```python
from build123d import *

# Parameters (mm, degrees)
BOX_W        = 100
BOX_H        = 32
BOX_DEPTH    = 52
SKETCH_W     = 100
SKETCH_H     = 25.7
POCKET_DEPTH = 5


with BuildPart() as part:
    # Box → Box (new body)
    with BuildSketch(Plane.XY):
        with Locations((50, 16)):
            Rectangle(BOX_W, BOX_H)
    extrude(amount=BOX_DEPTH)

    # Sketch → Pocket (cut)
    with BuildSketch(Plane.XZ):
        with Locations((50, 12.85)):
            Rectangle(SKETCH_W, SKETCH_H)
    extrude(amount=-POCKET_DEPTH, mode=Mode.SUBTRACT)


solid = part.part
```
Geometry: final body of the model. Coordinates: model frame, mm. A direction names the side the tool comes from. Coordinates: 2 decimals unless noted, no trailing zeros. Loops run counter-clockwise (first coordinate to the right, second up) from the corner with the lowest first, then second, coordinate; pieces in that order, holes last. Notation, with made-up numbers: (43, 29.5) -> (51, 29.5) arc R34 cw to (51, 59.5) -> close; hole circle Ø4 at (34, -21.5). An arc over 180 degrees is marked (long way). Use a Markdown table: item, result. Add a question column.
(1) Section query A-A, the plane x = 16. Return loops of the section in (y, z).
(2) Line query: line 1 along Z through (x, y) = (5, 3.5); line 2 along Y through (x, z) = (88, 5). Output: solid intervals per line, ascending.
(3) Pin query (flat end, axial travel): pin 1 Ø7.5 at (x, z) = (72.5, 11) entering from -Y. Return the tip coordinate at first contact, or that it passes through.
(4) Section query B-B, the plane z = 14.5. Return loops of the section in (x, y), plus the area to 3 significant figures.
(5) Access query for faces 1 (the flat face through (49, 5, 13)), 2 (the flat face through (49, 0, 39)). Directions: +Z, -Z, +X, -X, +Y, -Y. A direction counts if a zero-diameter tool reaches every point of the face in a straight line with its end or side. Return the directions, or none.
Answer:
| question | item | result |
|---|---|---|
| 1 | outline | (0, 25.7) -> (5, 25.7) -> (5, 0) -> (32, 0) -> (32, 52) -> (0, 52) -> close |
| 2 | line 1 | z = 25.7 to 52 |
| 2 | line 2 | y = 5 to 32 |
| 3 | pin 1 | stops at y = 5 |
| 4 | outline | (0, 5) -> (100, 5) -> (100, 32) -> (0, 32) -> close |
| 4 | area | 2,700 mm^2 |
| 5 | face 1 | -Z, +X, -X, -Y |
| 5 | face 2 | +Z, -Z, +X, -X, -Y |
